For this review, take the finished solid that the model builds, in its own axes (mm). A direction names the side the tool comes from. Give positions to 0.01 mm unless a question says otherwise; leave off trailing zeros. Write each loop counter-clockwise with the first axis right and the second up, starting at its lowest first coordinate (ties: lowest second). Pieces come first, ordered by that corner, then holes.
Q1. Insertion check: P1, Ø5, axis at x = 4, y = 2, coming from the +Z side; P2, Ø0.6, axis at x = -10, y = -1.5, coming from the -Z side; P3, Ø5, axis at x = -7, z = -6, coming from the -Y side. Each pin has a flat end and moves straight along its axis. Give the tip position at first contact, or say it passes through.
Q2. We need section C-C (z = -25). Write out the cut boundary in (x, y).
Q3. For line 1 (X direction, y = 4, z = -49); line 2 (Z direction, x = -1.25, y = 8.5); line 3 (Z direction, x = -1, y = 7.25), list the stretches that pass through material, from the lowest coordinate up.
Q4. Machinability: for faces 1 (the cylindrical face through (5.47, -1.01, -52.52)), 2 (the flat face through (8, -2, -49)), 3 (the flat face through (9, -1, -45)), 4 (the flat face through (-9, -1, -53)), which of the approach directions +Z, -Z, +X, -X, +Y, -Y give a long, thin tool a straight path to every point of the face, cutting with its end or side? Answer none if there is none.
Q5. We need section B-B (y = 5). Write out the cut boundary in (x, z), then the cut area to 3 significant figures.
Q6. Mouldability with a two-part tool opening along X and no side actions: class faces 5 (the cylindrical face through (6, -1, -49)), 6 (the cylindrical face through (-0.258, 4.93, 11.747)), 7 (the flat face through (-11.75, 5, -31)) as released by +X, released by -X, zero draft, split by the parting line, or undercut.
Q7. We need section A-A (z = -49). Write out the cut boundary in (x, y).
```python
from build123d import *
from build123d.topology import SkipClean

# Parameters (mm, degrees)
SKETCH1_R           = 3
SKETCH1_R_2         = 6.75
BOSS_EXTRUDE1_DEPTH = 10
BOSS_EXTRUDE2_START = 2
SKETCH2_W           = 23.5
SKETCH2_H           = 8
SKETCH2_R           = 3
BOSS_EXTRUDE2_DEPTH = 2
CHAMFER1_SIZE       = 3
SKETCH3_R           = 6
CUT_EXTRUDE1_DEPTH  = 2
FILLET1_R           = 1


with BuildPart() as part:
    # Sketch1 → Boss-Extrude1 (new body)
    with BuildSketch(Plane(origin=(0, 0, 0), x_dir=(1, 0, 0), z_dir=(0, 1, 0))):
        with BuildLine():
            Line((-11.75, 64), (-11.75, 0))
            ThreePointArc((-11.75, 0), (0, -11.75), (11.75, 0))
            Line((11.75, 0), (11.75, 64))
            Line((11.75, 64), (-11.75, 64))
        make_face()
        with Locations(Location((0, 49, 0), (0, 0, 270))):
            Circle(SKETCH1_R, mode=Mode.SUBTRACT)
        with Locations(Location((0, 0, 0), (0, 0, 270))):
            Circle(SKETCH1_R_2, mode=Mode.SUBTRACT)
    extrude(amount=BOSS_EXTRUDE1_DEPTH)

    # Sketch2 → Boss-Extrude2 (add)
    with SkipClean():  # the faces are left unmerged after this step: merging them gives an invalid solid
        with BuildSketch(Plane.XZ.offset(BOSS_EXTRUDE2_START)):
            with Locations((0, -49)):
                Rectangle(SKETCH2_W, SKETCH2_H)
            with Locations(Location((0, -49, 0), (0, 0, 270))):
                Circle(SKETCH2_R, mode=Mode.SUBTRACT)
        extrude(amount=-BOSS_EXTRUDE2_DEPTH)

    # Chamfer1
    chamfer1_edges = [part.edges().sort_by_distance(p)[0] for p in [
        (-11.75, 5, -64),
        (11.75, 5, -64),
    ]]
    chamfer(chamfer1_edges, length=CHAMFER1_SIZE)

    # Sketch3 → Cut-Extrude1 (cut)
    with BuildSketch(Plane.XZ.offset(2)):
        with Locations((0, -49)):
            Circle(SKETCH3_R)
    extrude(amount=-CUT_EXTRUDE1_DEPTH, mode=Mode.SUBTRACT)

    # Fillet1
    fillet1_edges = [part.edges().sort_by_distance(p)[0] for p in [
        (4.472135955, -1, -53),
        (-4.472135955, -1, -53),
        (4.472135955, -1, -45),
        (-4.472135955, -1, -45),
    ]]
    fillet(fillet1_edges, radius=FILLET1_R)


solid = part.part
```
Computed:
1. P1: stops at z = 11.65
1. P2: stops at z = -53
1. P3: stops at y = 0
2. outline: (-11.75, 0) - (11.75, 0) - (11.75, 10) - (-11.75, 10) - close
3. line 1: x = -11.75 to -3, 3 to 11.75
3. line 2: z = -64 to -51.73, -46.27 to -6.63, 6.63 to 11.68
3. line 3: z = -64 to -51.83, -46.17 to -6.68, 6.68 to 11.71
4. face 1: -Y
4. face 2: +Z, -Z, +X, -X, -Y
4. face 3: +Z, +X, -X, -Y
4. face 4: -Z, +X, -X, -Y
5. outline: (-11.75, -61) - (-8.75, -64) - (8.75, -64) - (11.75, -61) - (11.75, 0) arc R11.75 ccw to (-11.75, 0) - close; hole circle Ø13.5 at (0, 0); hole circle Ø6 at (0, -49)
5. area: 1,540 mm2
6. face 5: undercut
6. face 6: split by the parting line
6. face 7: released by -X
7. outline: (-11.75, -2) - (-6, -2) - (-6, 0) - (-3, 0) - (-3, 10) - (-11.75, 10) - close; (3, 0) - (6, 0) - (6, -2) - (11.75, -2) - (11.75, 10) - (3, 10) - close
